```python
from build123d import *

# Parameters (mm, degrees)
EXTRUDE_THIN1_DEPTH = 444.5
FILLET1_R           = 1.27


with BuildPart() as part:
    # Sketch1 → Extrude-Thin1 (new body)
    with BuildSketch(Plane.XY):
        with BuildLine():
            Line((0, 0), (-3.175, 0))
            ThreePointArc((-3.175, 0), (-3.702847988, 4.644874913), (-6.360025415, 8.491028131))
            ThreePointArc((-6.360025415, 8.491028131), (-8.643825609, 11.839848435), (-9.028393687, 15.875))
            Line((-9.028393687, 15.875), (-12.7, 15.875))
            Line((-12.7, 15.875), (-12.7, 44.45))
            Line((-12.7, 44.45), (0, 44.45))
            Line((0, 44.45), (0, 43.18))
            Line((0, 43.18), (-11.43, 43.18))
            Line((-11.43, 43.18), (-11.43, 17.145))
            Line((-11.43, 17.145), (-7.371031325, 17.145))
            ThreePointArc((-7.371031325, 17.145), (-7.668334251, 13.001809097), (-5.522110789, 9.445386071))
            ThreePointArc((-5.522110789, 9.445386071), (-2.789162607, 5.757129719), (-1.820706321, 1.27))
            Line((-1.820706321, 1.27), (0, 1.27))
            Line((0, 1.27), (0, 0))
        make_face()
    extrude(amount=-EXTRUDE_THIN1_DEPTH)

    # Fillet1
    fillet1_edges = [part.edges().sort_by_distance(p)[0] for p in [
        (-7.371031325, 17.145, -222.25),
        (-3.175, 0, -222.25),
        (-12.7, 15.875, -222.25),
        (-12.7, 44.45, -222.25),
    ]]
    fillet(fillet1_edges, radius=FILLET1_R)


solid = part.part
```
Geometry check sheet. Reference: the model listing, model coordinates, mm. A direction names the side the tool comes from. Give positions to 0.01 mm unless a question says otherwise; leave off trailing zeros. Order: outer loops, then holes, each group sorted by start corner. A loop starts at its lowest first (then second) coordinate and runs counter-clockwise, first axis right, second up.
1. Section check B-B, the plane y = 23.5. Enter the section's corners in (x, z).
2. Release check for a two-part mould opening along Y. For faces 3 (the face through (-6, 44.45, -219)), 4 (the face through (-2.82, 5.82, -219.14)), 5 (the face through (-12.7, 30, -219)) record: pulls with the +Y half, pulls with the -Y half, needs draft (parallel to the pull), parting line crosses it, or undercut.
3. Thickness scan on L1, parallel to Y at x = -1.75, z = -227; L2, parallel to Y at x = -11.25, z = -271 (3 decimals); L3, parallel to X at y = 34.5, z = -162.5. Record the ranges inside material, lowest first.
4. Section check A-A, the plane z = -299. Enter the section's corners in (x, y) (3 decimals), and give its area (3 significant figures).
5. Access from +Z, -Z, +X, -X, +Y, -Y to the whole of each face (thin tool, end or side, straight path). Record for faces 1 (the face through (-11.43, 30, -219)), 2 (the face through (-3.92, 5.18, -219.14)).
6. Gauge pin test, flat ends, axial feed: pin 1 Ø1 at (x, z) = (-7, -362.5) entering from -Y; pin 2 Ø2 at (y, z) = (37, -144.5) entering from +X; pin 3 Ø6 at (x, z) = (-10, -398.5) entering from -Y. Record the tip position at first contact, or that the pin passes through.
Values follow:
1. outline: (-12.7, -444.5) - (-11.43, -444.5) - (-11.43, 0) - (-12.7, 0) - close
2. face 3: pulls with the +Y half
2. face 4: undercut
2. face 5: needs draft
3. L1: y = 0 to 1.27, 43.18 to 44.45
3. L2: y = 15.875 to 17.145, 43.18 to 44.45
3. L3: x = -12.7 to -11.43
4. outline: (-12.7, 17.145) arc R1.27 ccw to (-11.43, 15.875) - (-9.028, 15.875) arc R8.136 ccw to (-6.36, 8.491) arc R9.609 cw to (-3.091, 1.27) arc R1.27 ccw to (-1.821, 0) - (0, 0) - (0, 1.27) - (-1.821, 1.27) arc R10.879 ccw to (-5.522, 9.445) arc R6.866 cw to (-7.774, 15.677) arc R1.27 ccw to (-9.028, 17.145) - (-11.43, 17.145) - (-11.43, 43.18) - (0, 43.18) - (0, 44.45) - (-11.43, 44.45) arc R1.27 ccw to (-12.7, 43.18) - close
4. area: 78.8 mm2
5. face 1: +Z, -Z, +X
5. face 2: +Z, -Z, -X, -Y
6. pin 1: stops at y = 8.62
6. pin 2: stops at x = -11.43
6. pin 3: stops at y = 9.12
